from build123d import *

# Parameters (mm, degrees)
BOSS_EXTRUDE1_DEPTH = 15
SKETCH2_R           = 1.7
CUT_EXTRUDE1_DEPTH  = 15


with BuildPart() as part:
    # Sketch1 → Boss-Extrude1 (new body)
    with BuildSketch(Plane(origin=(0, 0, 0), x_dir=(1, 0, 0), z_dir=(0, 1, 0))):
        with BuildLine():
            Line((0, 7.7), (0, 17.7))
            Line((0, 17.7), (-3, 17.7))
            Line((-3, 17.7), (-10, 14.909160565))
            Line((-10, 14.909160565), (-10, -15.090839435))
            Line((-10, -15.090839435), (-3, -17.7))
            Line((-3, -17.7), (0, -17.7))
            Line((0, -17.7), (0, -7.7))
            ThreePointArc((0, -7.7), (-7.7, 0), (0, 7.7))
        make_face()
    extrude(amount=BOSS_EXTRUDE1_DEPTH)

    # Sketch2 → Cut-Extrude1 (cut)
    with BuildSketch(Plane.ZY.offset(10)):
        with Locations((-11.909160565, 7.5)):
            Circle(SKETCH2_R)
        with Locations((11.909160565, 7.5)):
            Circle(SKETCH2_R)
    extrude(amount=-CUT_EXTRUDE1_DEPTH, mode=Mode.SUBTRACT)


solid = part.part
The model under review builds one solid part; all positions refer to its coordinate system, in mm. Coordinates: 2 decimals unless noted, no trailing zeros. Loops run counter-clockwise (first coordinate to the right, second up) from the corner with the lowest first, then second, coordinate; pieces in that order, holes last. Notation, with made-up numbers: (40, 69.25) -> (63, 69.25) arc R26 cw to (63, 104.25) -> close; hole circle Ø4 at (10, 0). An arc over 180 degrees is marked (long way). Use a Markdown table: item, result. Add a question column.
1. To check wall thickness, follow line 1 (Y direction, x = -6.75, z = 12); line 2 (Z direction, x = -5, y = 1.75); line 3 (Y direction, x = -1, z = 11.5). State the ranges of each line that lie inside material, in increasing order.
2. Add section B-B on y = 12.5. Write out the cut boundary in (x, z), plus the area to 3 significant figures.
3. Add section A-A on x = -1. Write out the cut boundary in (y, z), plus the area to 3 significant figures.
4. Add section C-C on y = 7.5. Write out the cut boundary in (x, z), plus the area to 3 significant figures.
5. Clearance check with flat-ended pins moving along their axes: pin 1 Ø5 at (x, y) = (-6, 10.5) entering from -Z; pin 2 Ø2 at (x, y) = (-7, 5) entering from +Z. State where each tip first meets the part, or that it passes through.
6. Draft analysis for pull direction Z (two halves, no side actions). For faces 1 (the face through (-5.07, 7.57, 10.21)), 2 (the face through (-5.07, 6.85, -10.34)), 3 (the face through (-1, 7, -17.7)), 4 (the face through (-10, 7, 0)), state which applies: pulls with the +Z half, pulls with the -Z half, needs draft (parallel to the pull), parting line crosses it, or undercut.
7. Add section D-D on z = 0. Write out the cut boundary in (x, y), plus the area to 3 significant figures.
Returned:
| question | item | result |
|---|---|---|
| 1 | line 1 | y = 0 to 5.8, 9.2 to 15 |
| 1 | line 2 | z = -16.9 to -5.86, 5.86 to 16.95 |
| 1 | line 3 | y = 0 to 5.85, 9.15 to 15 |
| 2 | outline | (-10, -14.91) -> (-3, -17.7) -> (0, -17.7) -> (0, -7.7) arc R7.7 cw to (0, 7.7) -> (0, 17.7) -> (-3, 17.7) -> (-10, 15.09) -> close |
| 2 | area | 242 mm² |
| 3 | outline | (0, -17.7) -> (15, -17.7) -> (15, -7.63) -> (0, -7.63) -> close; (0, 7.63) -> (15, 7.63) -> (15, 17.7) -> (0, 17.7) -> close; hole circle Ø3.4 at (7.5, -11.91); hole circle Ø3.4 at (7.5, 11.91) |
| 3 | area | 284 mm² |
| 4 | outline | (-10, -14.91) -> (-3, -17.7) -> (0, -17.7) -> (0, -13.61) -> (-10, -13.61) -> close; (-10, -10.21) -> (0, -10.21) -> (0, -7.7) arc R7.7 cw to (0, 7.7) -> (0, 10.21) -> (-10, 10.21) -> close; (-10, 13.61) -> (0, 13.61) -> (0, 17.7) -> (-3, 17.7) -> (-10, 15.09) -> close |
| 4 | area | 174 mm² |
| 5 | pin 1 | stops at z = -17.5 |
| 5 | pin 2 | stops at z = 16.58 |
| 6 | face 1 | undercut |
| 6 | face 2 | undercut |
| 6 | face 3 | pulls with the -Z half |
| 6 | face 4 | needs draft |
| 7 | outline | (-10, 0) -> (-7.7, 0) -> (-7.7, 15) -> (-10, 15) -> close |
| 7 | area | 34.5 mm² |
